Check sheet for the modelled part. Datum: model origin and axes. Units: mm. A direction names the side the tool comes from. Give positions to 0.01 mm unless a question says otherwise; leave off trailing zeros. Write each loop counter-clockwise with the first axis right and the second up, starting at its lowest first coordinate (ties: lowest second). Pieces come first, ordered by that corner, then holes.
Autodesk Inventor part; units mm, degrees
ref_plane "YZ Plane" through (0, 0, 0) normal (1, 0, 0) x (0, 1, 0)
ref_plane "XZ Plane" through (0, 0, 0) normal (0, 1, 0) x (-1, 0, 0)
ref_plane "XY Plane" through (0, 0, 0) normal (0, 0, 1) x (1, 0, 0)
sketch "Sketch1" plane through (0, 0, 0) normal (0, 1, 0) x (-1, 0, 0)
  circle A0 centre (0, 0) radius 37.5
  dimension "d0" = 75
extrude "Extrusion1" add sketch "Sketch1" along normal blind 12
sketch "Sketch3" plane through (0, 0, 0) normal (0, -1, 0) x (1, 0, 0)
  line L0 (41, 17.5) -> (-41, 17.5)
  line L1 (-41, 17.5) -> (-41, -17.5)
  line L2 (-41, -17.5) -> (41, -17.5)
  line L3 (41, -17.5) -> (41, 17.5)
  point P0 (0, 0)
  point P1 (41, 0)
  point P2 (0, -17.5)
  dimension "d6" = 82
  dimension "d7" = 35
extrude "Extrusion3" add sketch "Sketch3" against normal blind 4
sketch "Sketch4" plane through (0, 0, 0) normal (0, -1, 0) x (1, 0, 0)
  line L0 (-45, -2.625) -> (45, -2.625)
  line L1 (45, -2.625) -> (45, 2.625)
  line L2 (45, 2.625) -> (-45, 2.625)
  line L3 (-45, 2.625) -> (-45, -2.625)
  point P0 (0, 0)
  point P1 (-45, 0)
  point P2 (0, 2.625)
  dimension "d10" = 90
  dimension "d11" = 5.25
extrude "Extrusion4" add sketch "Sketch4" against normal blind 4
sketch "Sketch2" plane through (0, 12, 0) normal (0, 1, 0) x (1, 0, 0)
  circle A0 centre (0, 0) radius 33
  dimension "d3" = 66
extrude "Extrusion2" cut sketch "Sketch2" against normal blind 11
sketch "Sketch5" plane through (0, 1, 0) normal (0, 1, 0) x (1, 0, 0)
  circle A0 centre (0, 0) radius 4.1
  dimension "d14" = 8.2
extrude "Extrusion5" cut sketch "Sketch5" against normal through all
sketch "Sketch6" plane through (0, 12, 0) normal (0, 1, 0) x (1, 0, 0)
  line L0 (-23.4141, 14.0625) -> (-31.1923, 21.8407)
  line L1 (-31.1923, 21.8407) -> (-21.9999, 31.0331)
  line L2 (-21.9999, 31.0331) -> (-14.2217, 23.2549)
  line L3 (-14.2217, 23.2549) -> (-23.4141, 14.0625)
  line L4 (0, 0) -> (-32.7126, 0) construction
  line L5 (0, 0) -> (0, 33) construction
  circle A0 centre (0, 0) radius 33 construction
  circle A1 centre (0, 0) radius 37.5 construction
  dimension "d17" = 11
  dimension "d18" = 13
extrude "Extrusion6" cut sketch "Sketch6" against normal through all
properties part number "SnackClock_exterior_final"
1) Access from +Z, -Z, +X, -X, +Y, -Y to the whole of each face (thin tool, end or side, straight path). Record for faces 5 (the flat face through (0, 1, 7)), 6 (the flat face through (41, 2, 10)), 7 (the flat face through (43, 2, -2.625)), 8 (the flat face through (-43, 2, 2.625)).
2) Gauge pin test, flat ends, axial feed: pin 1 (1 mm diameter, centred on x = -18, z = -17.5, fed in from +Y); pin 2 (1.2 mm diameter, centred on x = -43.5, y = 2, fed in from -Z) (3 decimals); pin 3 (3 mm diameter, centred on y = 5, z = -28.5, fed in from -X). Record the tip position at first contact, or that the pin passes through.
3) Sectioned sample at B-B on x = 0. Record the boundary of the cut face in (y, z).
4) Sectioned sample at A-A on z = 0. Record the boundary of the cut face in (x, y), then the cut area to 3 significant figures.
5) Scan lines: L1, parallel to X at y = 8.25, z = 0; L2, parallel to X at y = 0.35, z = 0. Record each from-to range of solid material in increasing order.
6) Draft check along X on faces 1 (the flat face through (-18.754, 0.507, -18.723)), 2 (the cylindrical face through (37.376, 5.916, 3.049)), 3 (the flat face through (45, 2, 0)), 4 (the flat face through (39, 4, 0)). Enter one of: +X half, -X half, draft (parallel to the pull), parting line (faces both ways), or undercut.
7) Sectioned sample at C-C on x = -35. Record the boundary of the cut face in (y, z), then the cut area to 3 significant figures.
8) Sectioned sample at D-D on y = 6. Record the boundary of the cut face in (x, z), then the cut area to 3 significant figures.
Answers below:
1. face 5: +Y
1. face 6: +Z, +X, +Y, -Y
1. face 7: -Z, +X, +Y, -Y
1. face 8: +Z, -X, +Y, -Y
2. pin 1: stops at y = 1
2. pin 2: stops at z = -2.625
2. pin 3: stops at x = -20.97
3. outline: (0, -37.5) - (12, -37.5) - (12, -33) - (1, -33) - (1, -4.1) - (0, -4.1) - close; (0, 4.1) - (1, 4.1) - (1, 33) - (12, 33) - (12, 37.5) - (0, 37.5) - close
4. outline: (-45, 0) - (-4.1, 0) - (-4.1, 1) - (-33, 1) - (-33, 12) - (-37.5, 12) - (-37.5, 4) - (-45, 4) - close; (4.1, 0) - (45, 0) - (45, 4) - (37.5, 4) - (37.5, 12) - (33, 12) - (33, 1) - (4.1, 1) - close
4. area: 226 mm2
5. L1: x = -37.5 to -33, 33 to 37.5
5. L2: x = -45 to -4.1, 4.1 to 45
6. face 1: undercut
6. face 2: parting line
6. face 3: +X half
6. face 4: draft
7. outline: (0, -17.5) - (4, -17.5) - (4, -13.46) - (12, -13.46) - (12, 13.46) - (4, 13.46) - (4, 17.5) - (0, 17.5) - close
7. area: 355 mm2
8. outline: (-30.78, -21.43) - (-27.54, -18.19) arc R33 cw (long way) to (-18.38, -27.41) - (-21.61, -30.65) arc R37.5 ccw (long way) to start
8. area: 938 mm2
